```python
from build123d import *

# Parameters (mm, degrees)
SKETCH1_R           = 2.38125
BOSS_EXTRUDE1_DEPTH = 2


with BuildPart() as part:
    # Sketch1 → Boss-Extrude1 (new, symmetric)
    with BuildSketch(Plane(origin=(0, 0, 0), x_dir=(0, 0, -1), z_dir=(1, 0, 0))):
        with BuildLine():
            Line((-60.839919999, -25.371860345), (-36.087520647, -25.371860345))
            Line((-36.087520647, -25.371860345), (-26.022794648, -20.390042329))
            Line((-26.022794648, -20.390042329), (2.985497353, -6.031575768))
            ThreePointArc((2.985497353, -6.031575768), (6.578628627, 1.419417511), (0.23290188, 6.72598375))
            Line((0.23290188, 6.72598375), (-43.515144264, 6.72598375))
            Line((-43.515144264, 6.72598375), (-56.419454373, 3.818772093))
            ThreePointArc((-56.419454373, 3.818772093), (-56.573650174, 3.11024955), (-56.625400227, 2.386991318))
            Line((-56.625400227, 2.386991318), (-56.625400227, -13.559221537))
            ThreePointArc((-56.625400227, -13.559221537), (-56.966991368, -14.831463057), (-57.899887224, -15.761510537))
            ThreePointArc((-57.899887224, -15.761510537), (-61.267882579, -19.98604889), (-60.839919999, -25.371860345))
        make_face()
        with Locations((-54.236184525, -22.137211246)):
            Circle(SKETCH1_R, mode=Mode.SUBTRACT)
        with Locations((-50.410128911, 1.079375692)):
            Circle(SKETCH1_R, mode=Mode.SUBTRACT)
        with BuildLine():
            ThreePointArc((-38.916021454, 0.318688833), (-38.085451708, 1.633557707), (-36.568397511, 1.976008906))
            Line((-36.568397511, 1.976008906), (-19.797694446, -0.914638547))
            Line((-19.797694446, -0.914638547), (-21.730897843, -12.13052726))
            Line((-21.730897843, -12.13052726), (-40.504072916, -8.894727872))
            Line((-40.504072916, -8.894727872), (-38.916021454, 0.318688833))
        make_face(mode=Mode.SUBTRACT)
        Circle(SKETCH1_R, mode=Mode.SUBTRACT)
    extrude(amount=BOSS_EXTRUDE1_DEPTH, both=True)


solid = part.part
```
Can you work these out from the model? Positions are in its coordinate system, mm. A direction names the side the tool comes from. Coordinates: 2 decimals unless noted, no trailing zeros. Loops run counter-clockwise (first coordinate to the right, second up) from the corner with the lowest first, then second, coordinate; pieces in that order, holes last. Notation, with made-up numbers: (40, 58.25) - (87, 58.25) arc R17 cw to (87, 88.25) - close; hole circle Ø3 at (44.5, -31). An arc over 180 degrees is marked (long way). Answer as CSV lines item,"result". Start each with the question number.
1) Suppose I cut it at A-A (x = 1.4). Please give me the cut outline in (y, z).
2) Which directions (+Z, -Z, +X, -X, +Y, -Y) give clear straight access to the entire face, cutting with the end or side of a thin tool? Please do faces 5 (the flat face through (0, -5, 56.625)), 6 (the cylindrical face through (0.028, -19.912, 61.245)), 7 (the flat face through (0.028, -10.535, 30.986)).
3) Suppose I cut it at B-B (y = -3). Please give me the cut outline in (x, z).
4) Thinking about a two-plate mould opening in Y: for faces 1 (the flat face through (-2, -13, 28)), 2 (the cylindrical face through (0.028, 3.12, 56.572)), 3 (the cylindrical face through (0.028, 1.621, 38.104)), 4 (the cylindrical face through (-0.03, 0.17, 48.21)), which applies, pulls with the +Y half, pulls with the -Y half, needs draft (parallel to the pull), parting line crosses it, or undercut?
5) I need wall thicknesses on line 1 (Z direction, x = -0.05, y = -2); line 2 (Z direction, x = -1.25, y = 2.5); line 3 (Y direction, x = 1.6, z = 50). Which ranges of each line are inside material? Lowest first, please. Write a range as from..to.
6) Suppose I cut it at C-C (y = -19). Please give me the cut outline in (x, z).
7) For pin 1 (4 mm diameter, centred on y = 0, z = 0, fed in from +X); pin 2 (1.2 mm diameter, centred on x = -0.5, y = -3, fed in from +Z); pin 3 (5.5 mm diameter, centred on y = -22.14, z = 54.24, fed in from +X), each with a flat end and sliding along its axis, tell me the tip position at first contact or that it passes through.
Check result:
1,outline,"(-25.37, 36.09) - (-6.03, -2.99) arc R6.73 ccw to (6.73, -0.23) - (6.73, 43.52) - (3.82, 56.42) arc R5.08 ccw to (2.39, 56.63) - (-13.56, 56.63) arc R2.54 cw to (-15.76, 57.9) arc R7.35 ccw to (-25.37, 60.84) - close; hole circle Ø4.76 at (-22.14, 54.24); hole (-12.13, 21.73) - (-0.91, 19.8) - (1.98, 36.57) arc R2.03 ccw to (0.32, 38.92) - (-8.89, 40.5) - close; hole circle Ø4.76 at (0, 0); hole circle Ø4.76 at (1.08, 50.41)"
2,face 5,"+Z, +X, -X, +Y"
2,face 6,"+Z, +X, -X"
2,face 7,"+X, -X"
3,outline,"(-2, -6.02) - (2, -6.02) - (2, 20.16) - (-2, 20.16) - close; (-2, 39.49) - (2, 39.49) - (2, 56.63) - (-2, 56.63) - close"
4,face 1,"needs draft"
4,face 2,"pulls with the +Y half"
4,face 3,"undercut"
4,face 4,"undercut"
5,line 1,"z = -6.43..-1.29, 1.29..19.98, 39.32..56.63"
5,line 2,"z = -6.25..48.5, 52.32..56.62"
5,line 3,"y = -25.37..-1.27, 3.43..5.27"
6,outline,"(-2, 23.21) - (2, 23.21) - (2, 60.89) - (-2, 60.89) - close"
7,pin 1,"passes through"
7,pin 2,"stops at z = 56.63"
7,pin 3,"stops at x = 2"
